Autodesk Inventor part; units mm, degrees
ref_plane "YZ Plane" through (0, 0, 0) normal (1, 0, 0) x (0, 1, 0)
ref_plane "XZ Plane" through (0, 0, 0) normal (0, 1, 0) x (-1, 0, 0)
ref_plane "XY Plane" through (0, 0, 0) normal (0, 0, 1) x (1, 0, 0)
sketch "Sketch1" plane through (0, 0, 0) normal (0, 1, 0) x (-1, 0, 0)
  line L0 (0, 0) -> (0, -40)
  line L1 (0, 0) -> (40, 0) construction
  line L2 (0, 0) -> (-40, 0)
  line L3 (-6, -40) -> (-6, -6)
  line L4 (-6, -6) -> (-40, -6)
  line L5 (-40, 0) -> (-40, -6)
  line L6 (0, -40) -> (-6, -40)
  line L7 (-40, -6) -> (-6, -40)
  dimension "d0" = 40
  dimension "d1" = 90
  dimension "d2" = 40
  dimension "d3" = 6
extrude "Extrusion1" add sketch "Sketch1" along normal blind 3
sketch "Sketch2" plane through (0, 3, 0) normal (0, 1, 0) x (1, 0, 0)
  line L0 (0, 40) -> (0, 0)
  line L1 (0, 0) -> (0, 40)
  line L2 (0, 0) -> (40, 0)
  line L3 (40, 0) -> (0, 0)
  line L4 (6, 40) -> (6, 0)
  line L5 (40, 6) -> (6, 6)
  line L6 (40, 6) -> (6, 40)
  line L7 (40, 6) -> (40, 0)
  line L8 (6, 40) -> (0, 40)
  dimension "d6" = 6
extrude "Extrusion2" add sketch "Sketch2" along normal blind 20 contours L8 L4 L2 L0 | L4 L5 L7 L2
sketch "Sketch3" plane through (6, 3, -6) normal (1, 0, 0) x (0, 0, -1)
  line L0 (34, 20) -> (-6, 20)
  line L1 (-6, 20) -> (4, 20)
  line L2 (4, 20) -> (4, 10)
  line L3 (4, 10) -> (24, 10) construction
  line L4 (4, 7) -> (24, 7)
  line L5 (24, 13) -> (4, 13)
  arc A0 (4, 13) -> (4, 7) centre (4, 10) ccw
  arc A1 (24, 7) -> (24, 13) centre (24, 10) ccw
  point P0 (-6, -3)
  point P1 (14, 10)
  dimension "d9" = 10
  dimension "d10" = 10
  dimension "d11" = 20
  dimension "d12" = 6
extrude "Extrusion3" cut sketch "Sketch3" against normal blind 20
sketch "Sketch4" plane through (40, 3, -6) normal (0, 0, -1) x (-1, 0, 0)
  line L0 (10, 20) -> (10, 10)
  line L1 (10, 10) -> (30, 10) construction
  line L2 (10, 7) -> (30, 7)
  line L3 (30, 13) -> (10, 13)
  arc A0 (10, 13) -> (10, 7) centre (10, 10) ccw
  arc A1 (30, 7) -> (30, 13) centre (30, 10) ccw
  line L4 (40, -3) -> (40, 20)
  line L5 (0, 20) -> (34, 20)
  point P0 (20, 10)
  dimension "d16" = 10
  dimension "d17" = 20
  dimension "d18" = 6
  dimension "d35" = 10
  dimension "d36" = 13
extrude "Extrusion4" cut sketch "Sketch4" against normal blind 20
fillet "Fillet1" radius 2 3 edges at (0, 11.5, 0) (40, 11.5, 0) (0, 11.5, -40)
fillet "Fillet2" radius 2 2 edges at (23, 23, -6) (6, 23, -23)
fillet "Fillet3" radius 2 11 edges at (39.4142, 23, -0.5858) (40, 23, -3) (40, 22.4142, -5.4142) (40, 12, -6) (0.5858, 23, -0.5858) (0, 23, -20) (0.5858, 23, -39.4142) (3, 23, -40) (5.4142, 22.4142, -40) (6, 12, -40) (20, 23, 0)
fillet "Fillet4" radius 2 7 edges at (0.5858, 0, -39.4142) (4, 0, -40) (0.5858, 0, -0.5858) (20, 0, 0) (39.4142, 0, -0.5858) (40, 0, -4) (0, 0, -20)
properties part number "RightAngle_Bracket"
Read the model definition and answer for the solid it produces. Units are mm, in the model's axes. A direction names the side the tool comes from. Coordinates: 2 decimals unless noted, no trailing zeros. Loops run counter-clockwise (first coordinate to the right, second up) from the corner with the lowest first, then second, coordinate; pieces in that order, holes last.
Q1. The part is cut by section D-D on y = 8.5. Write down the section's boundary in (x, z).
Q2. The mould has two halves that part along X. Classify faces 1 (the face through (3, 13, -7)), 2 (the face through (20, 16, -3)), 3 (the face through (39.4, 0.57, -4.29)): +X half, -X half, draft (parallel to the pull), parting line (faces both ways), or undercut.
Q3. Which of the six approach directions +Z, -Z, +X, -X, +Y, -Y give full straight-line access (tool end or side, diameter ignored) to faces 4 (the face through (14, 3, -18)), 5 (the face through (40, 11, -3)), 6 (the face through (20, 10, -3)), 7 (the face through (3, 13, -33)), 8 (the face through (39.4, 22.43, -3.01))?
Q4. The part is cut by section B-B on x = 11.5. Write down the section's boundary in (y, z).
Q5. Each of these flat-tipped pins is pushed along its axis until it touches: pin 1 Ø6 at (x, y) = (8.5, 15.5) entering from +Z; pin 2 Ø1 at (x, y) = (25.5, 2.5) entering from -Z; pin 3 Ø1.5 at (x, y) = (35, 19.5) entering from -Z; pin 4 Ø18 at (x, z) = (29, -17) entering from +Y. Where does it stop, or does it pass through?
Q6. The part is cut by section C-C on y = 13. Write down the section's boundary in (x, z), and give its area (3 significant figures).
Q7. Consider probe 1 along Z at (x, y) = (14.5, 9.75); probe 2 along X at (y, z) = (21, -12.5); probe 3 along Y at (x, z) = (12.5, -23). Determine where each line is inside the solid, lowest interval first.
Q8. The part is cut by section A-A on z = -23. Write down the section's boundary in (x, y), and give its area (3 significant figures).
Results below:
1. outline: (0, -38) arc R2 ccw to (2, -40) - (4, -40) arc R2 ccw to (6, -38) - (6, -6) - (38, -6) arc R2 ccw to (40, -4) - (40, -2) arc R2 ccw to (38, 0) - (2, 0) arc R2 ccw to (0, -2) - close
2. face 1: draft
2. face 2: undercut
2. face 3: +X half
3. face 4: -Z, +X, +Y
3. face 5: +Z, -Z, +X, +Y, -Y
3. face 6: +Z, -Z
3. face 7: +X, -X
3. face 8: +Z, -Z, +X, +Y
4. outline: (0, -34.5) - (3, -34.5) - (3, -6) - (10, -6) - (10, 0) - (2, 0) arc R2 ccw to (0, -2) - close; (16, -6) - (21, -6) arc R2 ccw to (23, -4) - (23, -2) arc R2 ccw to (21, 0) - (16, 0) - close
5. pin 1: stops at z = 0
5. pin 2: stops at z = -21
5. pin 3: stops at z = -6
5. pin 4: stops at y = 3
6. outline: (0, -38) arc R2 ccw to (2, -40) - (4, -40) arc R2 ccw to (6, -38) - (6, -33) - (0, -33) - close; (0, -7) - (6, -7) - (6, -6) - (7, -6) - (7, 0) - (2, 0) arc R2 ccw to (0, -2) - close; (33, -6) - (38, -6) arc R2 ccw to (40, -4) - (40, -2) arc R2 ccw to (38, 0) - (33, 0) - close
6. area: 128 mm2
7. probe 1: z = -6 to 0
7. probe 2: x = 0 to 6
7. probe 3: y = 0 to 3
8. outline: (0, 2) arc R2 ccw to (2, 0) - (23, 0) - (23, 3) - (6, 3) - (6, 10) - (0, 10) - close; (0, 16) - (6, 16) - (6, 21) arc R2 ccw to (4, 23) - (2, 23) arc R2 ccw to (0, 21) - close
8. area: 150 mm2
